```python
from build123d import *

# Parameters (mm, degrees)
SKETCH1_R                      = 17.125
SKETCH1_R_2                    = 11
BASE_EXTRUDE_DEPTH             = 5
SK_RET_5_TAL_DEPTH             = 2837.452108268
SKETCH2_OUTSIDE_W              = 3414.424
SKETCH2_OUTSIDE_H              = 1500.924
BORTSK_RING_AF_BUKKESTOP_DEPTH = 5
BUKKESTOP_FARINA_DEPTH         = 5


with BuildPart() as part:
    # Sketch1 → Base-Extrude (new body)
    with BuildSketch(Plane.XY):
        with BuildLine():
            Line((0, 450.25), (0, 311.805149274))
            ThreePointArc((0, 311.805149274), (-2.719685229, 297.307627743), (-10.508906528, 284.781540969))
            Line((-10.508906528, 284.781540969), (-94.490164622, 193.132080081))
            ThreePointArc((-94.490164622, 193.132080081), (-95.432087377, 191.931880335), (-96.180469124, 190.602360622))
            Line((-96.180469124, 190.602360622), (-134.781265361, 107.822685955))
            ThreePointArc((-134.781265361, 107.822685955), (-135.215178753, 106.728141402), (-135.517434537, 105.590182681))
            Line((-135.517434537, 105.590182681), (-154.559858359, 11.993679344))
            ThreePointArc((-154.559858359, 11.993679344), (-152.504537753, 3.672946714), (-144.760611313, 0))
            Line((-144.760611313, 0), (17, 0))
            ThreePointArc((17, 0), (19.121320344, -0.878679656), (20, -3))
            Line((20, -3), (20, -17.334351162))
            ThreePointArc((20, -17.334351162), (19.242605724, -19.327017609), (17.352853621, -20.313527948))
            Line((17.352853621, -20.313527948), (-148.861908023, -40))
            Line((-148.861908023, -40), (-135.517434537, -105.590182681))
            ThreePointArc((-135.517434537, -105.590182681), (-135.215178753, -106.728141402), (-134.781265361, -107.822685955))
            Line((-134.781265361, -107.822685955), (-96.180469124, -190.602360622))
            ThreePointArc((-96.180469124, -190.602360622), (-95.432087377, -191.931880335), (-94.490164622, -193.132080081))
            Line((-94.490164622, -193.132080081), (-10.508906528, -284.781540969))
            ThreePointArc((-10.508906528, -284.781540969), (-2.719685229, -297.307627743), (0, -311.805149274))
            Line((0, -311.805149274), (0, -450.25))
            ThreePointArc((0, -450.25), (-0.878679656, -452.371320344), (-3, -453.25))
            Line((-3, -453.25), (-2584.097644203, -453.25))
            ThreePointArc((-2584.097644203, -453.25), (-2585.818373512, -452.707456133), (-2586.916722065, -451.27606043))
            Line((-2586.916722065, -451.27606043), (-2625.631918795, -344.906931626))
            ThreePointArc((-2625.631918795, -344.906931626), (-2626.368590965, -343.327133059), (-2627.368400571, -341.899256963))
            Line((-2627.368400571, -341.899256963), (-2775.320888862, -165.576347508))
            ThreePointArc((-2775.320888862, -165.576347508), (-2778.793852416, -159.560998181), (-2780, -152.720595315))
            Line((-2780, -152.720595315), (-2780, -22.342329219))
            ThreePointArc((-2780, -22.342329219), (-2780.635383686, -20.496092591), (-2782.272393125, -19.431901719))
            Line((-2782.272393125, -19.431901719), (-2797.727606875, -15.568098281))
            ThreePointArc((-2797.727606875, -15.568098281), (-2799.364616314, -14.503907409), (-2800, -12.657670781))
            Line((-2800, -12.657670781), (-2800, -3))
            ThreePointArc((-2800, -3), (-2799.121320344, -0.878679656), (-2797, 0))
            Line((-2797, 0), (-2792.062257748, 0))
            ThreePointArc((-2792.062257748, 0), (-2789.427026365, -0.750817072), (-2787.583225666, -2.777777778))
            ThreePointArc((-2787.583225666, -2.777777778), (-2783.087011135, -4.894412835), (-2780, -1))
            Line((-2780, -1), (-2780, 0))
            Line((-2780, 0), (-2780, 152.720595315))
            ThreePointArc((-2780, 152.720595315), (-2778.793852416, 159.560998181), (-2775.320888862, 165.576347508))
            Line((-2775.320888862, 165.576347508), (-2627.368400571, 341.899256963))
            ThreePointArc((-2627.368400571, 341.899256963), (-2626.368590965, 343.327133059), (-2625.631918795, 344.906931626))
            Line((-2625.631918795, 344.906931626), (-2586.916722065, 451.27606043))
            ThreePointArc((-2586.916722065, 451.27606043), (-2585.818373512, 452.707456133), (-2584.097644203, 453.25))
            Line((-2584.097644203, 453.25), (-3, 453.25))
            ThreePointArc((-3, 453.25), (-0.878679656, 452.371320344), (0, 450.25))
        make_face()
        with Locations((-147, 154.75)):
            Circle(SKETCH1_R, mode=Mode.SUBTRACT)
        with Locations(Location((-147, -154.75, 0), (0, 0, 180))):
            Circle(SKETCH1_R, mode=Mode.SUBTRACT)
        with Locations((-250, 57)):
            Circle(SKETCH1_R_2, mode=Mode.SUBTRACT)
        with Locations((-350, 57)):
            Circle(SKETCH1_R_2, mode=Mode.SUBTRACT)
        with Locations(Location((-250, -57, 0), (0, 0, 180))):
            Circle(SKETCH1_R_2, mode=Mode.SUBTRACT)
        with Locations(Location((-350, -57, 0), (0, 0, 180))):
            Circle(SKETCH1_R_2, mode=Mode.SUBTRACT)
    extrude(amount=BASE_EXTRUDE_DEPTH)

    # Sketch5 → Skåret 5 tal (cut, through all)
    with BuildSketch(Plane.XY.offset(5)):
        with BuildLine():
            Line((-2579.25, -414.25), (-2573, -414.25))
            ThreePointArc((-2573, -414.25), (-2570.878679656, -415.128679656), (-2570, -417.25))
            Line((-2570, -417.25), (-2570, -423.25))
            ThreePointArc((-2570, -423.25), (-2570.878679656, -425.371320344), (-2573, -426.25))
            Line((-2573, -426.25), (-2575.5, -426.25))
            ThreePointArc((-2575.5, -426.25), (-2580.25, -431), (-2575.5, -435.75))
            Line((-2575.5, -435.75), (-2571, -435.75))
            ThreePointArc((-2571, -435.75), (-2570.292893219, -436.042893219), (-2570, -436.75))
            Line((-2570, -436.75), (-2570, -437.25))
            ThreePointArc((-2570, -437.25), (-2570.292893219, -437.957106781), (-2571, -438.25))
            Line((-2571, -438.25), (-2575.5, -438.25))
            ThreePointArc((-2575.5, -438.25), (-2582.75, -431), (-2575.5, -423.75))
            Line((-2575.5, -423.75), (-2573.5, -423.75))
            ThreePointArc((-2573.5, -423.75), (-2572.792893219, -423.457106781), (-2572.5, -422.75))
            Line((-2572.5, -422.75), (-2572.5, -417.75))
            ThreePointArc((-2572.5, -417.75), (-2572.792893219, -417.042893219), (-2573.5, -416.75))
            Line((-2573.5, -416.75), (-2579.25, -416.75))
            ThreePointArc((-2579.25, -416.75), (-2579.957106781, -416.457106781), (-2580.25, -415.75))
            Line((-2580.25, -415.75), (-2580.25, -415.25))
            ThreePointArc((-2580.25, -415.25), (-2579.957106781, -414.542893219), (-2579.25, -414.25))
        make_face()
    extrude(amount=-SK_RET_5_TAL_DEPTH, mode=Mode.SUBTRACT)

    # Sketch2 outside → Bortskæring af bukkestop (cut)
    with BuildSketch(Plane.XY.offset(5)):
        with Locations((-1390, 0)):
            Rectangle(SKETCH2_OUTSIDE_W, SKETCH2_OUTSIDE_H)
        with BuildLine():
            Line((0, -453.25), (-2780, -453.25))
            Line((-2780, -453.25), (-2780, 453.25))
            Line((-2780, 453.25), (0, 453.25))
            Line((0, 453.25), (0, 58.791931013))
            Line((0, 58.791931013), (-145.038646448, 58.791931013))
            Line((-145.038646448, 58.791931013), (-156.594381353, 1.993679344))
            ThreePointArc((-156.594381353, 1.993679344), (-156.795134307, 0), (-156.594381353, -1.993679344))
            Line((-156.594381353, -1.993679344), (-145.038646448, -58.791931013))
            Line((-145.038646448, -58.791931013), (0, -58.791931013))
            Line((0, -58.791931013), (0, -453.25))
        make_face(mode=Mode.SUBTRACT)
    extrude(amount=-BORTSK_RING_AF_BUKKESTOP_DEPTH, mode=Mode.SUBTRACT)

    # Sketch6 → Bukkestop - Farina (add)
    with BuildSketch(Plane.XY.offset(5)):
        with BuildLine():
            Line((-2786.94787914, 5.638155725), (-2799.342020143, 10.149254129))
            ThreePointArc((-2799.342020143, 10.149254129), (-2799.819152044, 10.515370314), (-2800, 11.08894675))
            Line((-2800, 11.08894675), (-2800, 16))
            ThreePointArc((-2800, 16), (-2799.707106781, 16.707106781), (-2799, 17))
            Line((-2799, 17), (-2786, 17))
            ThreePointArc((-2786, 17), (-2784.585786438, 16.414213562), (-2784, 15))
            Line((-2784, 15), (-2784, 14.5))
            ThreePointArc((-2784, 14.5), (-2782, 12.5), (-2780, 14.5))
            Line((-2780, 14.5), (-2780, -14.5))
            ThreePointArc((-2780, -14.5), (-2782, -12.5), (-2784, -14.5))
            Line((-2784, -14.5), (-2784, -15))
            ThreePointArc((-2784, -15), (-2784.585786438, -16.414213562), (-2786, -17))
            Line((-2786, -17), (-2799, -17))
            ThreePointArc((-2799, -17), (-2799.707106781, -16.707106781), (-2800, -16))
            Line((-2800, -16), (-2800, -11.08894675))
            ThreePointArc((-2800, -11.08894675), (-2799.819152044, -10.515370314), (-2799.342020143, -10.149254129))
            Line((-2799.342020143, -10.149254129), (-2786.94787914, -5.638155725))
            ThreePointArc((-2786.94787914, -5.638155725), (-2783, 0), (-2786.94787914, 5.638155725))
        make_face()
        with BuildLine():
            Line((6.94787914, 5.638155725), (19.342020143, 10.149254129))
            ThreePointArc((19.342020143, 10.149254129), (19.819152044, 10.515370314), (20, 11.08894675))
            Line((20, 11.08894675), (20, 16))
            ThreePointArc((20, 16), (19.707106781, 16.707106781), (19, 17))
            Line((19, 17), (-19.424545303, 17))
            ThreePointArc((-19.424545303, 17), (-19.989696761, 16.946286447), (-20.534610691, 16.787069219))
            Line((-20.534610691, 16.787069219), (-149.930032595, -34.75))
            Line((-149.930032595, -34.75), (-140.774679121, -79.75))
            Line((-140.774679121, -79.75), (-20.650302992, -17.337873079))
            ThreePointArc((-20.650302992, -17.337873079), (-19.979067171, -17.085692127), (-19.267161546, -17))
            Line((-19.267161546, -17), (19, -17))
            ThreePointArc((19, -17), (19.707106781, -16.707106781), (20, -16))
            Line((20, -16), (20, -11.08894675))
            ThreePointArc((20, -11.08894675), (19.819152044, -10.515370314), (19.342020143, -10.149254129))
            Line((19.342020143, -10.149254129), (6.94787914, -5.638155725))
            ThreePointArc((6.94787914, -5.638155725), (3, 0), (6.94787914, 5.638155725))
        make_face()
    extrude(amount=-BUKKESTOP_FARINA_DEPTH)


solid = part.part
```
Can you work these out from the model? Positions are in its coordinate system, mm. A direction names the side the tool comes from. Round coordinates to 2 decimals unless told otherwise and drop trailing zeros. Answer in a Markdown table with one row per item.
Item 1: We'd pull the mould along Y, two halves only. Please class faces 4 (the flat face through (-1410, 6, 5)), 5 (the flat face through (-2702.38, 252.504, 2.465)), 6 (the flat face through (-81.55, -48.98, 2.54)): released by +Y, released by -Y, zero draft, split by the parting line, or undercut.
Answer block:
| item | result |
|---|---|
| face 4 | zero draft |
| face 5 | released by +Y |
| face 6 | undercut |
Item 2: If I drill on probe 1 along Y at (x, z) = (-250, 3.45); probe 2 along X at (y, z) = (-154.75, 1.45) (3 decimals); probe 3 along X at (y, z) = (-57, 2.45), over which ranges is the centre line in solid material (lowest first)?
Answer block:
| item | result |
|---|---|
| probe 1 | -453.25 to -68, -46 to 46, 68 to 453.25 |
| probe 2 | -2779.897 to -164.125, -129.875 to -112.899 |
| probe 3 | -2780 to -361, -339 to -261, -239 to -96.99 |
Item 3: Suppose I cut it at A-A, the plane z = 4.1. Give the number of separate pieces and of enclosed holes in the cut face, plus the area to 3 significant figures.
Answer block:
| item | result |
|---|---|
| separate pieces | 1 |
| enclosed holes | 7 |
| area | 2,400,000 mm² |
Item 4: Will these pins go through, and if not, where does the flat tip stop? P1, Ø2.5, axis at x = 6, z = 3, coming from the +Y side; P2, Ø2.5, axis at y = -379, z = 3, coming from the +X side; P3, Ø2.5, axis at y = -87, z = 2.5, coming from the -X side.
Answer block:
| item | result |
|---|---|
| P1 | y = 17 |
| P2 | x = 0 |
| P3 | x = -2780 |
Item 5: On a 3-axis mill with a long thin cutter (end or side, diameter ignored), from which of +Z, -Z, +X, -X, +Y, -Y can I reach the whole of each face in a straight line? I mean faces 1 (the flat face through (-84.33, -8.62, 2.54)), 2 (the flat face through (-53.1, -238.3, 2.5)), 3 (the flat face through (-2700.31, -254.97, 2.46)). Say none if no direction works.
Answer block:
| item | result |
|---|---|
| face 1 | +Z, -Z |
| face 2 | +Z, -Z, +X |
| face 3 | +Z, -Z, -X, -Y |
